The listing builds one solid part. Answer for the finished solid, in the listing's coordinates (mm). Give positions to 0.01 mm unless a question says otherwise; leave off trailing zeros. Loops run counter-clockwise (first coordinate to the right, second up) from the corner with the lowest first, then second, coordinate; pieces in that order, holes last. Notation, with made-up numbers: (55, -34.5) -> (72, -34.5) arc R27 ccw to (72, -3.5) -> close; hole circle Ø10 at (32, -10). An arc over 180 degrees is marked (long way). One line per question, with ' | ' between items. Start each with the question number.
from build123d import *

# Parameters (mm, degrees)
SKETCH_1_R      = 10
EXTRUDE_2_DEPTH = 10


with BuildPart() as part:
    # 草图1 → 凸台-拉伸2 (new body)
    with BuildSketch(Plane.XY):
        with BuildLine():
            ThreePointArc((20, 0), (0, 20), (-20, 0))
            Line((-20, 0), (-20, -100))
            Line((-20, -100), (20, -100))
            Line((20, -100), (20, 0))
        make_face()
        Circle(SKETCH_1_R, mode=Mode.SUBTRACT)
        with Locations((0, -54)):
            Circle(SKETCH_1_R, mode=Mode.SUBTRACT)
    extrude(amount=EXTRUDE_2_DEPTH)


solid = part.part
1. Determine the mould class of faces 1 (the flat face through (0, -100, 5)), 2 (the cylindrical face through (-2.17, -9.76, 4.93)), 3 (the flat face through (-20, -49, 5)), 4 (the cylindrical face through (-2.17, -63.76, 4.93)) for opening direction Y: released by +Y, released by -Y, zero draft, split by the parting line, or undercut.
2. The part is cut by section C-C (z = 3.75). Write down the section's boundary in (x, y).
3. Each of these flat-tipped pins is pushed along its axis until it touches: pin 1 Ø4 at (x, y) = (-4.5, -34.5) entering from -Z; pin 2 Ø16 at (x, y) = (0, 0) entering from +Z; pin 3 Ø5 at (x, z) = (-8.5, 6) entering from +Y. Where does it stop, or does it pass through?
4. The part is cut by section D-D (y = -7). Write down the section's boundary in (x, z).
5. The part is cut by section B-B (x = 0). Write down the section's boundary in (y, z).
6. Straight lines are drawn through the part: L1, parallel to Y at x = 0, z = 7.5; L2, parallel to Y at x = -2, z = 6.75; L3, parallel to X at y = -49, z = 4.25. For each, find the intervals that lie inside material, in ascending order.
7. The part is cut by section A-A (y = -54). Write down the section's boundary in (x, z).
Check sheet entries:
1) face 1: released by -Y | face 2: undercut | face 3: zero draft | face 4: undercut
2) outline: (-20, -100) -> (20, -100) -> (20, 0) arc R20 ccw to (-20, 0) -> close; hole circle Ø20 at (0, -54); hole circle Ø20 at (0, 0)
3) pin 1: stops at z = 0 | pin 2: passes through | pin 3: stops at y = 19.08
4) outline: (-20, 0) -> (-7.14, 0) -> (-7.14, 10) -> (-20, 10) -> close; (7.14, 0) -> (20, 0) -> (20, 10) -> (7.14, 10) -> close
5) outline: (-100, 0) -> (-64, 0) -> (-64, 10) -> (-100, 10) -> close; (-44, 0) -> (-10, 0) -> (-10, 10) -> (-44, 10) -> close; (10, 0) -> (20, 0) -> (20, 10) -> (10, 10) -> close
6) L1: y = -100 to -64, -44 to -10, 10 to 20 | L2: y = -100 to -63.8, -44.2 to -9.8, 9.8 to 19.9 | L3: x = -20 to -8.66, 8.66 to 20
7) outline: (-20, 0) -> (-10, 0) -> (-10, 10) -> (-20, 10) -> close; (10, 0) -> (20, 0) -> (20, 10) -> (10, 10) -> close
